Input: part model. Units: mm. Frame: model coordinates. A direction names the side the tool comes from. Coordinates: 2 decimals unless noted, no trailing zeros. Write each loop counter-clockwise with the first axis right and the second up, starting at its lowest first coordinate (ties: lowest second). Pieces come first, ordered by that corner, then holes. Notation, with made-up numbers: (85.25, 22.25) - (124.25, 22.25) arc R27 cw to (124.25, 39.25) - close; hole circle Ø9 at (77, -20). An arc over 180 degrees is marked (long way). Put each result on its own line as item: value. Start each with the question number.
1. Cut plane B-B, the plane x = 78. Return loops of the section in (y, z).
2. Line query: line 1 (X direction, y = 3.5, z = -1); line 2 (X direction, y = -6.5, z = -4.5); line 3 (Z direction, x = 73, y = -16.5). Output: solid intervals per line, ascending.
3. Access query for faces 5 (the flat face through (88.176, 22, 0)), 6 (the flat face through (93.129, 22, 0)), 7 (the cylindrical face through (11.8, 0.84, -10.05)). Directions: +Z, -Z, +X, -X, +Y, -Y. A direction counts if a zero-diameter tool reaches every point of the face in a straight line with its end or side. Return the directions, or none.
4. Pin query (flat end, axial travel): pin 1 (2.5 mm diameter, centred on x = 91.5, y = 20.5, fed in from +Z); pin 2 (1.5 mm diameter, centred on x = 68.5, y = -3.5, fed in from +Z); pin 3 (6 mm diameter, centred on x = 23.5, z = -16, fed in from +Y); pin 4 (5.5 mm diameter, centred on y = 22, z = 2, fed in from +X). Return the tip coordinate at first contact, or that it passes through.
5. Pull-direction query (Z, two-part tool) for faces 1 (the cylindrical face through (16.76, -0.89, 11.54)), 2 (the flat face through (10.3, 0, 13)), 3 (the cylindrical face through (19.021, 2.455, 0.545)), 4 (the flat face through (91, 21, 9.169)); classes: released by +Z, released by -Z, zero draft, split by the parting line, or undercut.
from build123d import *

# Parameters (mm, degrees)
BOSS_EXTRUDE1_DEPTH = 3.429
BOSS_EXTRUDE2_DEPTH = 2.4765
SKETCH7_R           = 1.4605
BOSS_EXTRUDE5_DEPTH = 6.9088
SKETCH8_R           = 2.7813
BOSS_EXTRUDE6_DEPTH = 2.9591


with BuildPart() as part:
    # Sketch1 → Revolve1 (revolve)
    with BuildSketch(Plane.XY, mode=Mode.PRIVATE) as revolve1_sk:
        Polygon((94.6404, 0), (94.6404, 19.9771), (23.9268, 19.9771), (20.1676, 16.42566681), (20.1676, 2.5146), (17.907, 2.5146), (17.907, 5.4864), (9.779, 5.4864), (9.779, 8.2804), (3.9116, 8.2804), (3.9116, 2.5146), (0, 2.5146), (0, 0), align=None)
    revolve(revolve1_sk.sketch.rotate(Axis((94.6404, 0, 0), (-1, 0, 0)), 90), axis=Axis((94.6404, 0, 0), (-1, 0, 0)))

    # Sketch3 → Boss-Extrude1 (add, symmetric)
    with BuildSketch(Plane(origin=(90.6526, 0, 0), x_dir=(0, 0, -1), z_dir=(1, 0, 0))):
        with BuildLine():
            Line((-9.7917, 18.985047302), (-9.157160583, 17.754743999))
            ThreePointArc((-9.157160583, 17.754743999), (0, -19.9771), (9.157160583, 17.754743999))
            Line((9.157160583, 17.754743999), (9.7917, 18.985047302))
            ThreePointArc((9.7917, 18.985047302), (0, 21.3614), (-9.7917, 18.985047302))
        make_face()
    extrude(amount=BOSS_EXTRUDE1_DEPTH, both=True)

    # Sketch4 → Boss-Extrude2 (add, symmetric)
    with BuildSketch(Plane(origin=(90.6526, 0, 0), x_dir=(0, 0, -1), z_dir=(1, 0, 0))):
        with BuildLine():
            Line((-9.1694, 19.293302299), (-9.1694, 22.442902299))
            ThreePointArc((-9.1694, 22.442902299), (0, 24.243798381), (9.1694, 22.442902299))
            Line((9.1694, 22.442902299), (9.1694, 19.293302299))
            ThreePointArc((9.1694, 19.293302299), (9.48180276, 19.141703852), (9.7917, 18.985047302))
            Line((9.7917, 18.985047302), (9.157160583, 17.754743999))
            ThreePointArc((9.157160583, 17.754743999), (0, 19.9771), (-9.157160583, 17.754743999))
            Line((-9.157160583, 17.754743999), (-9.7917, 18.985047302))
            ThreePointArc((-9.7917, 18.985047302), (-9.48180276, 19.141703852), (-9.1694, 19.293302299))
        make_face()
    extrude(amount=BOSS_EXTRUDE2_DEPTH, both=True)

    # Sketch7 → Boss-Extrude5 (add)
    with BuildSketch(Plane.ZY.offset(-20.1676)):
        with Locations((-12.7, 0)):
            Circle(SKETCH7_R)
        with Locations((12.7, 0)):
            Circle(SKETCH7_R)
    extrude(amount=BOSS_EXTRUDE5_DEPTH)

    # Sketch8 → Boss-Extrude6 (add)
    with BuildSketch(Plane.ZY.offset(-13.2588)):
        with Locations((12.7, 0)):
            Circle(SKETCH8_R)
        with Locations((-12.7, 0)):
            Circle(SKETCH8_R)
    extrude(amount=BOSS_EXTRUDE6_DEPTH)


solid = part.part
Report:
1. outline: circle Ø39.95 at (0, 0)
2. line 1: x = 3.91 to 17.91, 20.17 to 94.64
2. line 2: x = 3.91 to 9.78, 20.17 to 94.64
2. line 3: z = -11.26 to 11.26
3. face 5: -X, +Y
3. face 6: +X, +Y
3. face 7: -X
4. pin 1: stops at z = 9.26
4. pin 2: stops at z = 19.79
4. pin 3: stops at y = 15.14
4. pin 4: stops at x = 94.64
5. face 1: undercut
5. face 2: zero draft
5. face 3: undercut
5. face 4: released by +Z
